Geometry check sheet. Reference: the model listing, model coordinates, mm. A direction names the side the tool comes from. Round coordinates to 2 decimals unless told otherwise and drop trailing zeros. Write each loop counter-clockwise with the first axis right and the second up, starting at its lowest first coordinate (ties: lowest second). Pieces come first, ordered by that corner, then holes. Notation, with made-up numbers: (-9.5, 1.25) - (25.5, 1.25) arc R26 ccw to (25.5, 26.25) - close; hole circle Ø8 at (30, -15.75). An arc over 180 degrees is marked (long way). Return JSON: item names as keys, results as strings.
```python
from build123d import *

# Parameters (mm, degrees)
SKETCH1_W                                          = 69.85
SKETCH1_H                                          = 44.45
BOSS_EXTRUDE1_DEPTH                                = 9.525
CSK_FOR_10_FLAT_HEAD_MACHINE_SCREW_100_D           = 5.1054
CSK_FOR_10_FLAT_HEAD_MACHINE_SCREW_100_CSINK_D     = 9.779
CSK_FOR_10_FLAT_HEAD_MACHINE_SCREW_100_CSINK_ANGLE = 82
FILLET4_R                                          = 6.35
F_1_4_0_25_DIAMETER_HOLE1_D                        = 6.35
SKETCH10_W                                         = 15.875
SKETCH10_H                                         = 15.875
CUT_EXTRUDE2_DEPTH                                 = 3.175
FILLET5_R                                          = 6.35
FILLET5_OF_MIRROR2_R                               = 6.35
MIRROR3_START                                      = 6.35
MIRROR3_OUTLINE_R                                  = 3.175
MIRROR3_DEPTH                                      = 3.175


# Read off the part's stored shape, not the designer's step: Mirror3
with BuildPart() as part:
    # Sketch1 → Boss-Extrude1 (new body)
    with BuildSketch(Plane(origin=(0, 0, 0), x_dir=(1, 0, 0), z_dir=(0, 1, 0))):
        Rectangle(SKETCH1_W, SKETCH1_H)
    extrude(amount=BOSS_EXTRUDE1_DEPTH)

    # CSK for #10 Flat Head Machine Screw (100)1 (through all)
    with Locations(Plane(origin=(0, 0, 0), x_dir=(-1, 0, 0), z_dir=(0, -1, 0))):
        with Locations((0, 11.1125), (0, -11.1125)):
            CounterSinkHole(CSK_FOR_10_FLAT_HEAD_MACHINE_SCREW_100_D / 2, CSK_FOR_10_FLAT_HEAD_MACHINE_SCREW_100_CSINK_D / 2, counter_sink_angle=CSK_FOR_10_FLAT_HEAD_MACHINE_SCREW_100_CSINK_ANGLE)

    # Fillet4
    fillet4_edges = [part.edges().sort_by_distance(p)[0] for p in [
        (34.925, 4.7625, 22.225),
        (-34.925, 4.7625, 22.225),
        (-34.925, 4.7625, -22.225),
        (34.925, 4.7625, -22.225),
    ]]
    fillet(fillet4_edges, radius=FILLET4_R)

    # 1/4 (0.25) Diameter Hole1 (through all)
    with Locations(Plane(origin=(0, 0, 0), x_dir=(-1, 0, 0), z_dir=(0, -1, 0))):
        with Locations((-28.575, 15.875), (-28.575, -15.875)):
            f_1_4_0_25_diameter_hole1 = Hole(F_1_4_0_25_DIAMETER_HOLE1_D / 2)

    # Mirror1: 1/4 (0.25) Diameter Hole1 across plane
    add(f_1_4_0_25_diameter_hole1.mirror(Plane(origin=(0, 0, 0), x_dir=(0, 0, 1), z_dir=(1, 0, 0))), mode=Mode.SUBTRACT)

    # Sketch10 → Cut-Extrude2 (cut)
    with BuildSketch(Plane(origin=(0, 9.525, 0), x_dir=(1, 0, 0), z_dir=(0, 1, 0))):
        with Locations((-26.9875, 14.2875)):
            Rectangle(SKETCH10_W, SKETCH10_H)
    cut_extrude2 = extrude(amount=-CUT_EXTRUDE2_DEPTH, mode=Mode.SUBTRACT)

    # Fillet5
    fillet5_edges = [part.edges().sort_by_distance(p)[0] for p in [
        (-19.05, 7.9375, -6.35),
    ]]
    fillet(fillet5_edges, radius=FILLET5_R)

    # Mirror2: Cut-Extrude2 across plane
    add(cut_extrude2.mirror(Plane.XY), mode=Mode.SUBTRACT)

    # Fillet5 of Mirror2
    fillet5_of_mirror2_edges = [part.edges().sort_by_distance(p)[0] for p in [
        (-19.05, 7.9375, 6.35),
    ]]
    fillet(fillet5_of_mirror2_edges, radius=FILLET5_OF_MIRROR2_R)

    # Mirror3 outline → Mirror3 (cut)
    # profile 1 of 2: a face of its own
    with BuildSketch(Plane(origin=(0, 0, 0), x_dir=(1, 0, 0), z_dir=(0, 1, 0)).offset(MIRROR3_START)):
        with BuildLine():
            Line((25.4, 6.35), (34.925, 6.35))
            Line((34.925, 6.35), (34.925, 15.875))
            ThreePointArc((34.925, 15.875), (33.065128061, 20.365128061), (28.575, 22.225))
            Line((28.575, 22.225), (19.05, 22.225))
            Line((19.05, 22.225), (19.05, 12.7))
            ThreePointArc((19.05, 12.7), (20.909871939, 8.209871939), (25.4, 6.35))
        make_face()
        with Locations((28.575, 15.875)):
            Circle(MIRROR3_OUTLINE_R, mode=Mode.SUBTRACT)
    # profile 2 of 2: a face of its own
    with BuildSketch(Plane(origin=(0, 0, 0), x_dir=(1, 0, 0), z_dir=(0, 1, 0)).offset(MIRROR3_START)):
        with BuildLine():
            Line((34.925, -15.875), (34.925, -6.35))
            Line((34.925, -6.35), (25.4, -6.35))
            ThreePointArc((25.4, -6.35), (20.909871939, -8.209871939), (19.05, -12.7))
            Line((19.05, -12.7), (19.05, -22.225))
            Line((19.05, -22.225), (28.575, -22.225))
            ThreePointArc((28.575, -22.225), (33.065128061, -20.365128061), (34.925, -15.875))
        make_face()
        with Locations((28.575, -15.875)):
            Circle(MIRROR3_OUTLINE_R, mode=Mode.SUBTRACT)
    extrude(amount=MIRROR3_DEPTH, mode=Mode.SUBTRACT)


solid = part.part
```
(1) Release check for a two-part mould opening along Z. For faces 1 (the face through (33.11, 3.22, -20.32)), 2 (the face through (25.403, 3.219, 15.735)), 3 (the face through (-19.05, 8, -17)) record: pulls with the +Z half, pulls with the -Z half, needs draft (parallel to the pull), parting line crosses it, or undercut.
Response values:
{"face 1": "pulls with the -Z half", "face 2": "undercut", "face 3": "needs draft"}
(2) Section check A-A, the plane x = 0. Enter the section's corners in (y, z) (3 decimals).
Response values:
{"outline": "(0, -22.225) - (9.525, -22.225) - (9.525, -13.665) - (2.688, -13.665) - (0, -16.002) - close; (0, -6.223) - (2.688, -8.56) - (9.525, -8.56) - (9.525, 8.56) - (2.688, 8.56) - (0, 6.223) - close; (0, 16.002) - (2.688, 13.665) - (9.525, 13.665) - (9.525, 22.225) - (0, 22.225) - close"}
(3) Material ranges on line 1 along Z through (x, y) = (0, 6) (3 decimals); line 2 along X through (y, z) = (3.25, 11) (3 decimals); line 3 along Z through (x, y) = (0.5, 4.25) (3 decimals), recorded low to high. Write a range as [from, to].
Response values:
{"line 1": "z = [-22.225, -13.665], [-8.56, 8.56], [13.665, 22.225]", "line 2": "x = [-34.925, -2.55], [2.55, 34.925]", "line 3": "z = [-22.225, -13.616], [-8.609, 8.609], [13.616, 22.225]"}
(4) Section check B-B, the plane y = 1. Give the number of separate pieces and of enclosed holes in the cut face, plus the area to 3 significant figures.
Response values:
{"separate pieces": "1", "enclosed holes": "6", "area": "2,840 mm^2"}
(5) Gauge pin test, flat ends, axial feed: pin 1 (2.5 mm diameter, centred on y = 8.5, z = 16, fed in from -X); pin 2 (8 mm diameter, centred on x = -26.5, z = 15, fed in from +Y); pin 3 (1.6 mm diameter, centred on x = -32, y = 7.5, fed in from -Z). Record the tip position at first contact, or that the pin passes through.
Response values:
{"pin 1": "stops at x = -19.05", "pin 2": "stops at y = 6.35", "pin 3": "stops at z = -6.35"}
(6) Section check C-C, the plane x = 24. Enter the section's corners in (y, z) (3 decimals).
Response values:
{"outline": "(0, -22.225) - (6.35, -22.225) - (6.35, -6.506) - (9.525, -6.506) - (9.525, 6.506) - (6.35, 6.506) - (6.35, 22.225) - (0, 22.225) - close"}
(7) Access from +Z, -Z, +X, -X, +Y, -Y to the whole of each face (thin tool, end or side, straight path). Record for faces 4 (the face through (20.86, 7.92, -8.26)), 5 (the face through (25, 6.35, 14)), 6 (the face through (-27.1, 6.35, 12.6)).
Response values:
{"face 4": "-Z, +X, +Y", "face 5": "+Z, +X, +Y", "face 6": "+Z, -X, +Y"}
